Autodesk Inventor part; units mm, degrees
ref_plane "Work Plane1" through (29, 0, 0) normal (0, -1, 0) x (1, 0, 0)
ref_plane "YZ Plane" through (0, 0, 0) normal (1, 0, 0) x (0, 1, 0)
ref_plane "XZ Plane" through (0, 0, 0) normal (0, 1, 0) x (-1, 0, 0)
sketch "Sketch1" plane through (0, 0, 0) normal (0, 0, 1) x (1, 0, 0)
  line L0 (-0.1333, 0) -> (25, 0)
  line L1 (25, 0) -> (25, 4)
  line L2 (25, 4) -> (3.75, 4)
  line L3 (3.75, 4) -> (2.9831, 4)
  line L4 (2.9831, 4) -> (0, 4)
  line L5 (0, 4) -> (0, 7)
  line L6 (0, 7) -> (-4.4, 7)
  line L7 (-4.4, 7) -> (-4.4, 2.8868)
  line L8 (-4.4, 2.8868) -> (-1.8, 2.8868)
  line L9 (-1.8, 2.8868) -> (-0.1333, 0)
  line L10 (-10.28, 0) -> (30.88, 0)
  line L11 (0, -1.4) -> (0, 8.4)
  line L12 (3.75, 4) -> (0, 4) construction
  dimension "d1" = 21.25
  dimension "d2" = 0.7669
  dimension "d3" = 4.4
  dimension "d4" = 2.6
  dimension "d5" = 60
  dimension "d6" = 8
  dimension "d7" = 8
  dimension "d8" = 5.7735
  dimension "d9" = 14
  dimension "d26" = 25
revolve "Body" add sketch "Sketch1" angle 360 about axis through (-0.1333, 0, 0) along (1, 0, 0)
sketch "Sketch2" plane through (-4.4, 0, 0) normal (-1, 0, 0) x (0, 0, 1)
  circle A0 centre (0, 0) radius 2.8868
  line L0 (0, -9.8) -> (0, 9.8)
  line L1 (-9.8, 0) -> (9.8, 0)
  line L2 (2.8868, 0) -> (1.4434, -2.5)
  line L3 (1.4434, -2.5) -> (-1.4434, -2.5)
  line L4 (-1.4434, -2.5) -> (-2.8868, 0)
  line L5 (-2.8868, 0) -> (-1.4434, 2.5)
  line L6 (-1.4434, 2.5) -> (1.4434, 2.5)
  line L7 (1.4434, 2.5) -> (2.8868, 0)
extrude "Slot" add sketch "Sketch2" against normal up to next contours L7 A0 | A0 L2 | L6 L0 A0 | A0 L0 L3 | L0 L6 A0 | A0 L3 L0 | L4 A0 | A0 L5
fillet "Fillet1" radius 3.35 1 edges at (-4.4, -7, 0)
thread "Thread"
chamfer "Chamfer1" distance 0.7668 distance2 0.7668 1 edges at (25, -4, 0) measured on face at (25, -0.6859, 0.8072)
ref_plane "Work Plane1" through (29, 0, 0) normal (0, -1, 0) x (1, 0, 0)
fillet "Fillet2" radius 0.7 1 edges at (0, -4, 0)
equation "\"d1\" = GEL"
equation "\"d3\" = KOH"
equation "\"d4\" = INTI"
equation "\"d6\" = GD"
equation "\"d7\" = BDM"
equation "\"d8\" = 1.1547 * SW"
equation "\"d9\" = KOD"
equation "\"d26\" = NLG"
equation "\"d30\" = R"
equation "\"d17\" = RR"
equation "\"d13\" = GEL"
equation "\"d15\" = -0.5 * SPD + 0.5 * GD"
equation "\"d16\" = GUL"
equation "\"GD\" = NND"
equation "\"NLG\" = 25"
equation "\"GEL\" = 21.25"
equation "\"KOD\" = 14"
equation "\"KOH\" = 4.4"
equation "\"INTI\" = 2.6"
equation "\"GAL\" = 0.61345 * PTC"
equation "\"GUL\" = 0.61345 * PTC"
equation "\"BDM\" = NND"
equation "\"SW\" = 5"
equation "\"RR\" = 3.35"
equation "\"SPD\" = NND - 1.2269 * PTC"
equation "\"R\" = 0.7"
equation "\"TOA\" = 30deg"
equation "\"GD1\" = THREADDIA - 1.2269 * PTC"
equation "\"THREADDIA\" = 8"
equation "\"PTC\" = 1.25"
equation "\"NND\" = 8"
equation "\"KOH1\" = 1.05"
equation "\"E0\" = 5.723"
properties part number "PWTR-0073" material "Stainless Steel"
Verification items for the finished model (mm, model axes). A direction names the side the tool comes from. Round coordinates to 2 decimals unless told otherwise and drop trailing zeros. Write each loop counter-clockwise with the first axis right and the second up, starting at its lowest first coordinate (ties: lowest second). Pieces come first, ordered by that corner, then holes. Notation, with made-up numbers: (87.25, 23) -> (105.25, 23) arc R21 cw to (105.25, 39) -> close; hole circle Ø2 at (-8, 36). An arc over 180 degrees is marked (long way). Write each question's results on one line, items separated by ' | '.
Q1. Sectioned sample at A-A, the plane x = 11.5. Record the boundary of the cut face in (y, z).
Derived:
outline: circle Ø8 at (0, 0)
Q2. Thickness scan on probe 1 along Z at (x, y) = (12.25, 0); probe 2 along Z at (x, y) = (-1.75, 2); probe 3 along Y at (x, z) = (-1.75, -0.25). Record the ranges inside material, lowest first.
Derived:
probe 1: z = -4 to 4 | probe 2: z = -6.63 to -1.73, 1.73 to 6.63 | probe 3: y = -6.92 to -2.5, 2.5 to 6.92
Q3. Sectioned sample at B-B, the plane x = -0.75. Record the boundary of the cut face in (y, z).
Derived:
outline: circle Ø14 at (0, 0); hole circle Ø2.14 at (0, 0)
Q4. Draft check along Y on faces 1 (the face through (-4.4, -2, 2)), 2 (the face through (12.302, -0.867, 3.905)), 3 (the face through (-3.008, 1.268, 2.155)). Enter one of: released by +Y, released by -Y, zero draft, split by the parting line, or undercut.
Derived:
face 1: zero draft | face 2: split by the parting line | face 3: undercut
Q5. Go/stop test with flat-tipped pins: pin 1 Ø4 at (x, z) = (11, -2) entering from -Y; pin 2 Ø1 at (y, z) = (-4, 0) entering from -X; pin 3 Ø1.4 at (x, z) = (-2.5, 0.5) entering from +Y; pin 4 Ø4 at (x, y) = (9.5, -2.5) entering from +Z. Record where each tip stops, or that it passes through.
Derived:
pin 1: stops at y = -4 | pin 2: stops at x = -4.4 | pin 3: stops at y = 6.9 | pin 4: stops at z = 3.97
Q6. Access from +Z, -Z, +X, -X, +Y, -Y to the whole of each face (thin tool, end or side, straight path). Record for faces 4 (the face through (0, 1, -5)), 5 (the face through (-3.008, -1.233, 2.175)), 6 (the face through (-0.532, 6.466, 2.681)).
Derived:
face 4: +X | face 5: -X | face 6: +X, -X
